Can you work these out from the model? Positions are in its coordinate system, mm. Give positions to 0.01 mm unless a question says otherwise; leave off trailing zeros. Loops run counter-clockwise (first coordinate to the right, second up) from the corner with the lowest first, then second, coordinate; pieces in that order, holes last. Notation, with made-up numbers: (82.25, -12) - (126.25, -12) arc R22 ccw to (126.25, 8) - close; hole circle Ø3 at (7.25, 59). An arc over 180 degrees is marked (long way). Answer in a Markdown table with one row per item.
from build123d import *

# Parameters (mm, degrees)
BOSS_EXTRU_1_OUTLINE_R   = 50
BOSS_EXTRU_1_OUTLINE_W   = 5
BOSS_EXTRU_1_OUTLINE_H   = 5
BOSS_EXTRU_1_OUTLINE_R_2 = 1.5
BOSS_EXTRU_1_DEPTH       = 5
SKETCH4_R                = 2.8
CUT_EXTRUDE4_DEPTH       = 10
SKETCH5_R                = 40.5
CUT_EXTRUDE5_DEPTH       = 10


# Read off the part's stored shape, not the designer's step: Boss.-Extru.1
with BuildPart() as part:
    # Boss.-Extru.1 outline → Boss.-Extru.1 (new body)
    with BuildSketch(Plane.XY):
        Circle(BOSS_EXTRU_1_OUTLINE_R)
        Polygon((-37.262039705, -33.060254038), (-39.762039705, -28.730127019), (-35.431912686, -26.230127019), (-32.931912686, -30.560254038), align=None, mode=Mode.SUBTRACT)
        with Locations((-7.5, -46.3)):
            Rectangle(BOSS_EXTRU_1_OUTLINE_W, BOSS_EXTRU_1_OUTLINE_H, mode=Mode.SUBTRACT)
        with Locations((-40.096976195, -23.15)):
            Circle(BOSS_EXTRU_1_OUTLINE_R_2, mode=Mode.SUBTRACT)
        Polygon((-42.931912686, -13.239745962), (-40.431912686, -17.569872981), (-44.762039705, -20.069872981), (-47.262039705, -15.739745962), align=None, mode=Mode.SUBTRACT)
        with Locations((0, -46.3)):
            Circle(BOSS_EXTRU_1_OUTLINE_R_2, mode=Mode.SUBTRACT)
        with Locations((7.5, -46.3)):
            Rectangle(BOSS_EXTRU_1_OUTLINE_W, BOSS_EXTRU_1_OUTLINE_H, mode=Mode.SUBTRACT)
        Polygon((32.931912686, -30.560254038), (35.431912686, -26.230127019), (39.762039705, -28.730127019), (37.262039705, -33.060254038), align=None, mode=Mode.SUBTRACT)
        with Locations((40.096976195, -23.15)):
            Circle(BOSS_EXTRU_1_OUTLINE_R_2, mode=Mode.SUBTRACT)
        Polygon((47.262039705, -15.739745962), (44.762039705, -20.069872981), (40.431912686, -17.569872981), (42.931912686, -13.239745962), align=None, mode=Mode.SUBTRACT)
        Polygon((-47.262039705, 15.739745962), (-44.762039705, 20.069872981), (-40.431912686, 17.569872981), (-42.931912686, 13.239745962), align=None, mode=Mode.SUBTRACT)
        with Locations((-40.096976195, 23.15)):
            Circle(BOSS_EXTRU_1_OUTLINE_R_2, mode=Mode.SUBTRACT)
        Polygon((-32.931912686, 30.560254038), (-35.431912686, 26.230127019), (-39.762039705, 28.730127019), (-37.262039705, 33.060254038), align=None, mode=Mode.SUBTRACT)
        with Locations((-7.5, 46.3)):
            Rectangle(BOSS_EXTRU_1_OUTLINE_W, BOSS_EXTRU_1_OUTLINE_H, mode=Mode.SUBTRACT)
        Polygon((42.931912686, 13.239745962), (40.431912686, 17.569872981), (44.762039705, 20.069872981), (47.262039705, 15.739745962), align=None, mode=Mode.SUBTRACT)
        with Locations((40.096976195, 23.15)):
            Circle(BOSS_EXTRU_1_OUTLINE_R_2, mode=Mode.SUBTRACT)
        with Locations((0, 46.3)):
            Circle(BOSS_EXTRU_1_OUTLINE_R_2, mode=Mode.SUBTRACT)
        with Locations((7.5, 46.3)):
            Rectangle(BOSS_EXTRU_1_OUTLINE_W, BOSS_EXTRU_1_OUTLINE_H, mode=Mode.SUBTRACT)
        Polygon((37.262039705, 33.060254038), (39.762039705, 28.730127019), (35.431912686, 26.230127019), (32.931912686, 30.560254038), align=None, mode=Mode.SUBTRACT)
    extrude(amount=BOSS_EXTRU_1_DEPTH)

    # Sketch4 → Cut-Extrude4 (cut)
    with BuildSketch(Plane.XY.offset(5)):
        with Locations((-12.16449512, -45.398513836)):
            Circle(SKETCH4_R)
        with Locations((-45.398513836, 12.16449512)):
            Circle(SKETCH4_R)
        with Locations((12.16449512, 45.398513836)):
            Circle(SKETCH4_R)
        with Locations((45.398513836, -12.16449512)):
            Circle(SKETCH4_R)
    extrude(amount=-CUT_EXTRUDE4_DEPTH, mode=Mode.SUBTRACT)

    # Sketch5 → Cut-Extrude5 (cut)
    with BuildSketch(Plane.XY.offset(5)):
        Circle(SKETCH5_R)
    extrude(amount=-CUT_EXTRUDE5_DEPTH, mode=Mode.SUBTRACT)


solid = part.part
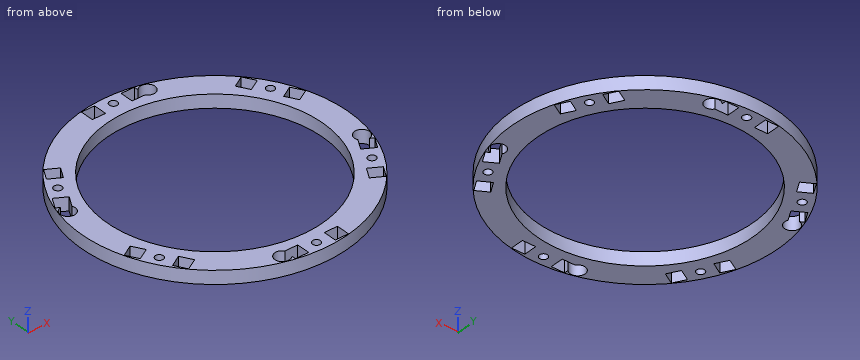
Q1. Imagine slicing it at A-A, the plane x = 0. Write out the boundary of the cut face in (y, z).
Checked values:
| item | result |
|---|---|
| outline | (-50, 0) - (-47.8, 0) - (-47.8, 5) - (-50, 5) - close; (-44.8, 0) - (-40.5, 0) - (-40.5, 5) - (-44.8, 5) - close; (40.5, 0) - (44.8, 0) - (44.8, 5) - (40.5, 5) - close; (47.8, 0) - (50, 0) - (50, 5) - (47.8, 5) - close |
Q2. Imagine slicing it at B-B, the plane y = 0. Write out the boundary of the cut face in (x, z).
Checked values:
| item | result |
|---|---|
| outline | (-50, 0) - (-40.5, 0) - (-40.5, 5) - (-50, 5) - close; (40.5, 0) - (50, 0) - (50, 5) - (40.5, 5) - close |
Q3. Imagine slicing it at C-C, the plane x = 18. Write out the boundary of the cut face in (y, z).
Checked values:
| item | result |
|---|---|
| outline | (-46.65, 0) - (-36.28, 0) - (-36.28, 5) - (-46.65, 5) - close; (36.28, 0) - (46.65, 0) - (46.65, 5) - (36.28, 5) - close |
Q4. Imagine slicing it at D-D, the plane y = 23.15. Write out the boundary of the cut face in (x, z).
Checked values:
| item | result |
|---|---|
| outline | (-44.32, 0) - (-41.6, 0) - (-41.6, 5) - (-44.32, 5) - close; (-38.6, 0) - (-33.23, 0) - (-33.23, 5) - (-38.6, 5) - close; (33.23, 0) - (38.6, 0) - (38.6, 5) - (33.23, 5) - close; (41.6, 0) - (44.32, 0) - (44.32, 5) - (41.6, 5) - close |
Q5. If I drill on line 1 (Y direction, x = 0, z = 3); line 2 (X direction, y = 30.5, z = 4.85); line 3 (Y direction, x = -5.5, z = 1.5), over which ranges is the centre line in solid material (lowest first)? Write a range as [from, to].
Checked values:
| item | result |
|---|---|
| line 1 | y = [-50, -47.8], [-44.8, -40.5], [40.5, 44.8], [47.8, 50] |
| line 2 | x = [-39.62, -38.74], [-32.97, -26.65], [26.65, 32.97], [38.74, 39.62] |
| line 3 | y = [-49.7, -48.8], [-43.8, -40.12], [40.12, 43.8], [48.8, 49.7] |
Q6. For pin 1 (1.5 mm diameter, centred on y = -26.5, z = 2, fed in from -X); pin 2 (2.5 mm diameter, centred on x = 8, z = 2.5, fed in from +Y); pin 3 (2.5 mm diameter, centred on y = -46, z = 2, fed in from +X), each with a flat end and sliding along its axis, tell me the tip position at first contact or that it passes through.
Checked values:
| item | result |
|---|---|
| pin 1 | stops at x = -42.86 |
| pin 2 | stops at y = 49.54 |
| pin 3 | stops at x = 22.3 |
